from build123d import *

# Parameters (mm, degrees)
SKETCH_2_R          = 7.5
EXTRUDE_1_DEPTH     = 127.5
SKETCH_3_R          = 7.5
REVOLVE_1_ANGLE     = 90
REVOLVE_2_OUTLINE_R = 7.5
REVOLVE_2_ANGLE     = 90
SKETCH_19_R         = 7.5
EXTRUDE_2_DEPTH     = 5
SKETCH_21_R         = 7.5
EXTRUDE_3_DEPTH     = 5
SKETCH_22_R         = 7.5
REVOLVE_3_ANGLE     = 90
SKETCH_23_R         = 7.5
REVOLVE_4_ANGLE     = 90
SKETCH_25_R         = 3.75
EXTRUDE_4_DEPTH     = 10
EXTRUDE_START       = 10
SKETCH_26_R         = 3.75
EXTRUDE_5_DEPTH     = 10


# Read off the part's stored shape, not the designer's step: Повернуть2
with BuildPart() as part:
    # Эскиз2 → Бобышка-Вытянуть1 (new body)
    with BuildSketch(Plane.XY):
        Circle(SKETCH_2_R)
    extrude(amount=EXTRUDE_1_DEPTH)

    # Эскиз3 → Повернуть1 (revolve)
    with BuildSketch(Plane.XY.offset(127.5)):
        with Locations(Location((0, 0, 0), (0, 0, 180))):
            Circle(SKETCH_3_R)
    revolve(axis=Axis((16, 0, 127.5), (0, 1, 0)), revolution_arc=REVOLVE_1_ANGLE)

    # Повернуть2 outline → Повернуть2 (revolve)
    with BuildSketch(Plane(origin=(16, 0, 0), x_dir=(0, 0, -1), z_dir=(1, 0, 0))):
        with Locations((16, 0)):
            Circle(REVOLVE_2_OUTLINE_R)
    revolve(axis=Axis((16, 0, 0), (0, 1, 0)), revolution_arc=REVOLVE_2_ANGLE)

    # Эскиз19 → Бобышка-Вытянуть2 (add)
    with BuildSketch(Plane(origin=(16, 0, 0), x_dir=(0, 0, -1), z_dir=(1, 0, 0))):
        with Locations((16, 0)):
            Circle(SKETCH_19_R)
    extrude(amount=EXTRUDE_2_DEPTH)

    # Эскиз21 → Бобышка-Вытянуть3 (add)
    with BuildSketch(Plane(origin=(16, 0, 0), x_dir=(0, 0, -1), z_dir=(1, 0, 0))):
        with Locations(Location((-143.5, 0, 0), (0, 0, 180))):
            Circle(SKETCH_21_R)
    extrude(amount=EXTRUDE_3_DEPTH)

    # Эскиз22 → Повернуть3 (revolve)
    with BuildSketch(Plane(origin=(21, 0, 0), x_dir=(0, 0, -1), z_dir=(1, 0, 0))):
        with Locations((16, 0)):
            Circle(SKETCH_22_R)
    revolve(axis=Axis((21, 0, 0), (0, -1, 0)), revolution_arc=REVOLVE_3_ANGLE)

    # Эскиз23 → Повернуть4 (revolve)
    with BuildSketch(Plane(origin=(21, 0, 0), x_dir=(0, 0, -1), z_dir=(1, 0, 0))):
        with Locations(Location((-143.5, 0, 0), (0, 0, 180))):
            Circle(SKETCH_23_R)
    revolve(axis=Axis((21, 0, 127.5), (0, 1, 0)), revolution_arc=REVOLVE_4_ANGLE)

    # Эскиз25 → Бобышка-Вытянуть4 (add)
    with BuildSketch(Plane.XY):
        with Locations((37, 0)):
            Circle(SKETCH_25_R)
    extrude(amount=EXTRUDE_4_DEPTH)

    # Эскиз26 → Бобышка-Вытянуть5 (add)
    with BuildSketch(Plane(origin=(0, 0, 127.5), x_dir=(-1, 0, 0), z_dir=(0, 0, -1)).offset(EXTRUDE_START)):
        with Locations(Location((-37, 0, 0), (0, 0, 180))):
            Circle(SKETCH_26_R)
    extrude(amount=-EXTRUDE_5_DEPTH)


solid = part.part
Check sheet for the modelled part. Datum: model origin and axes. Units: mm. A direction names the side the tool comes from. Coordinates: 2 decimals unless noted, no trailing zeros. Loops run counter-clockwise (first coordinate to the right, second up) from the corner with the lowest first, then second, coordinate; pieces in that order, holes last. Notation, with made-up numbers: (48.25, 66) -> (88.25, 66) arc R12 cw to (88.25, 81) -> close; hole circle Ø11 at (33.5, 32). An arc over 180 degrees is marked (long way). Write item = value, one per line. Start each with the question number.
1. Depth check by flat-ended pin: P1, Ø6, axis at x = 37.5, y = -1.5, coming from the +Z side; P2, Ø6, axis at x = 37, y = -1, coming from the -Z side; P3, Ø12, axis at x = 15.5, z = 77, coming from the -Y side; P4, Ø8, axis at y = 0.5, z = 57.5, coming from the +X side. Enter the tip coordinate at first touch or a pass-through.
2. Section check A-A on z = 3. Record the cut outline in (x, y), then the cut area to 3 significant figures.
3. Section check B-B on y = 0. Record the cut outline in (x, z).
4. Draft check along X on faces 3 (the flat face through (37, 0, 10)), 4 (the cylindrical face through (40.577, -1.126, 122.43)), 5 (the cylindrical face through (33.254, 0.165, 4.93)). Enter one of: released by +X, released by -X, zero draft, split by the parting line, or undercut.
5. Material ranges on line 1 (Z direction, x = 21.5, y = -0.5); line 2 (X direction, y = 0.25, z = 110); line 3 (Z direction, x = 10, y = 1.25), recorded low to high.
6. Tool access check on faces 1 (the flat face through (37, 0, 117.5)), 2 (the flat face through (40, 3, 127.5)). Record the directions out of +Z, -Z, +X, -X, +Y, -Y that give a thin tool (end or side, any length) a straight path to the whole face; none if there is none.
Responses:
q1.P1 = 146.63
q1.P2 = -19.53
q1.P3 = through
q1.P4 = 7.5
q2.outline = circle Ø15 at (0, 0); circle Ø7.5 at (37, 0)
q2.area = 221 mm2
q3.outline = (-7.5, 0) arc R23.5 ccw to (16, -23.5) -> (21, -23.5) arc R23.5 ccw to (44.5, 0) -> (40.75, 0) -> (40.75, 10) -> (33.25, 10) -> (33.25, 0) -> (29.5, 0) arc R8.5 cw to (21, -8.5) -> (16, -8.5) arc R8.5 cw to (7.5, 0) -> (7.5, 127.5) arc R8.5 cw to (16, 136) -> (21, 136) arc R8.5 cw to (29.5, 127.5) -> (33.25, 127.5) -> (33.25, 117.5) -> (40.75, 117.5) -> (40.75, 127.5) -> (44.5, 127.5) arc R23.5 ccw to (21, 151) -> (16, 151) arc R23.5 ccw to (-7.5, 127.5) -> close
q4.face_3 = zero draft
q4.face_4 = undercut
q4.face_5 = undercut
q5.line_1 = -23.48 to -8.5, 136 to 150.98
q5.line_2 = -7.5 to 7.5
q5.line_3 = -22.61 to -6.17, 133.67 to 150.11
q6.face_1 = +X, +Y, -Y
q6.face_2 = none
